Geometry check sheet. Reference: drawing and pictorial views, mm from the part's lowest x, y, z. Give positions to 0.01 mm unless a question says otherwise; leave off trailing zeros. Order: outer loops, then holes, each group sorted by start corner. A loop starts at its lowest first (then second) coordinate and runs counter-clockwise, first axis right, second up.
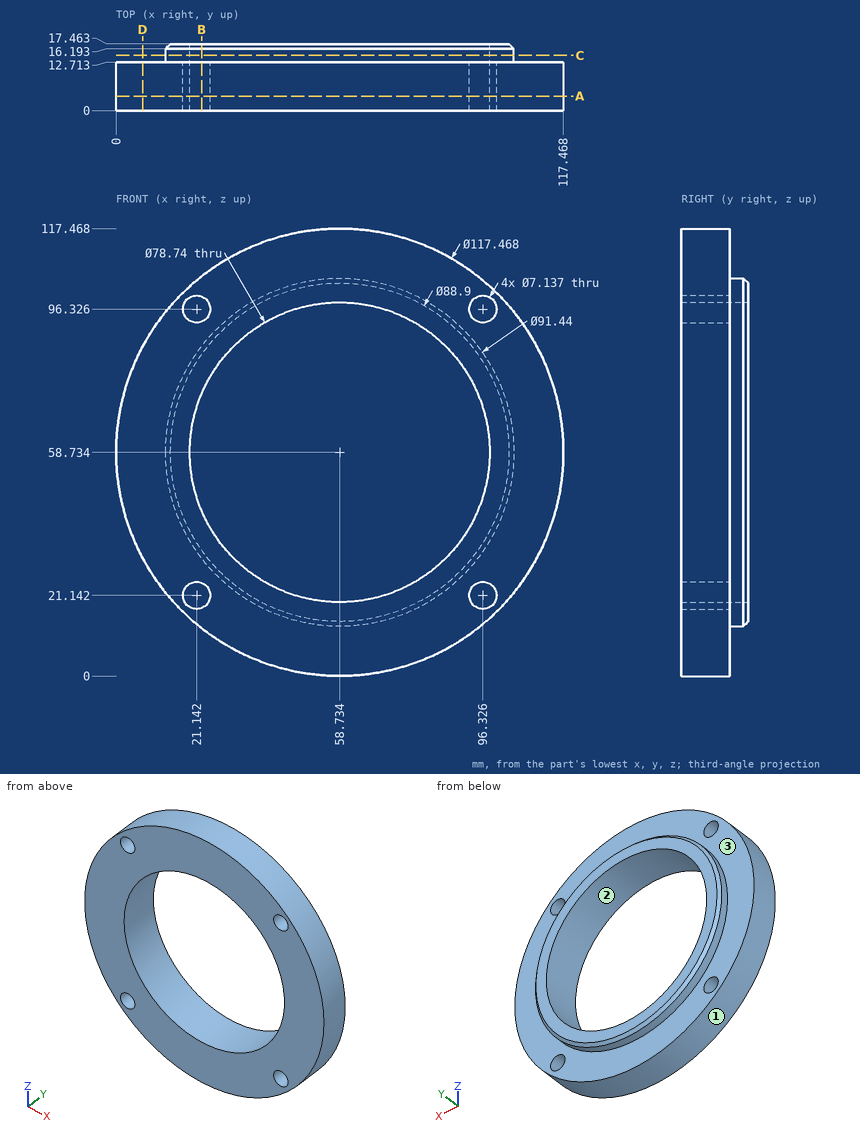
(1) Cross-section at B-B on x = 22.5. Count the separate pieces of the cut face and the enclosed holes in it, then the cut area to 3 significant figures.
Response values:
separate pieces: 4
enclosed holes: 0
area: 732 mm2
(2) Cross-section at C-C on y = 14.5. Enter the section's corners in (x, z) (1 decimal), then the cut area to 3 significant figures.
Response values:
outline: circle Ø91.4 at (58.7, 58.7); hole circle Ø78.7 at (58.7, 58.7)
area: 1,700 mm2
(3) Release check for a two-part mould opening along Z. For the marked faces 1, 2 and 3 record: released by +Z, released by -Z, zero draft, split by the parting line, or undercut.
Response values:
face 1: split by the parting line
face 2: undercut
face 3: zero draft
(4) Cross-section at A-A on y = 3.75. Enter the section's corners in (x, z) (1 decimal), then the cut area to 3 significant figures.
Response values:
outline: circle Ø117.5 at (58.7, 58.7); hole circle Ø7.1 at (21.1, 21.1); hole circle Ø7.1 at (21.1, 96.3); hole circle Ø78.7 at (58.7, 58.7); hole circle Ø7.1 at (96.3, 21.1); hole circle Ø7.1 at (96.3, 96.3)
area: 5,810 mm2
(5) Material ranges on L1, parallel to Y at x = 54, z = 108.5; L2, parallel to X at y = 15.5, z = 59.5; L3, parallel to X at y = 9.25, z = 29 (1 decimal), recorded low to high.
Response values:
L1: y = 0 to 12.71
L2: x = 13.02 to 19.37, 98.1 to 104.45
L3: x = 8.1 to 32.9, 84.5 to 109.4
(6) Cross-section at D-D on x = 7. Enter the section's corners in (y, z), then the cut area to 3 significant figures.
Response values:
outline: (0, 30.93) - (12.71, 30.93) - (12.71, 86.54) - (0, 86.54) - close
area: 707 mm2
(7) Gauge pin test, flat ends, axial feed: pin 1 Ø3 at (y, z) = (10, 66) entering from -X; pin 2 Ø2 at (x, y) = (80.5, 5) entering from +Z (1 decimal); pin 3 Ø5.5 at (x, z) = (96.33, 96.33) entering from -Y; pin 4 Ø2 at (x, y) = (13, 10.5) entering from +Z (1 decimal). Record the tip position at first contact, or that the pin passes through.
Response values:
pin 1: stops at x = 0.28
pin 2: stops at z = 113.7
pin 3: passes through
pin 4: stops at z = 96.8
